Here's how the part is built. I have some questions about the finished solid (model axes, mm). Round coordinates to 2 decimals unless told otherwise and drop trailing zeros. Loops run counter-clockwise (first coordinate to the right, second up) from the corner with the lowest first, then second, coordinate; pieces in that order, holes last. Notation, with made-up numbers: M 86,68 L 99,68 A18 ccw 99,103 Z; hole C -23.75,-33.5 d5. An arc over 180 degrees is marked long. One line per question, with ' | ' between items. Start each with the question number.
```python
from build123d import *

# Parameters (mm, degrees)
SKETCH3_R           = 1.4224
SKETCH3_W           = 6.35
SKETCH3_H           = 6.35
SKETCH3_W_2         = 11.938
SKETCH3_H_2         = 23.114
SKETCH3_W_3         = 101.6
SKETCH3_H_3         = 76.2
BOSS_EXTRUDE1_DEPTH = 6.35
FILLET1_R           = 10.16
FILLET2_R           = 27.94


with BuildPart() as part:
    # Sketch3 → Boss-Extrude1 (new body)
    with BuildSketch(Plane(origin=(0, 0, 0), x_dir=(1, 0, 0), z_dir=(0, 1, 0))):
        with BuildLine():
            Line((182.88, 0), (0, 0))
            Line((0, 0), (0, 262.339276313))
            Line((0, 262.339276313), (182.88, 262.339276313))
            Line((182.88, 262.339276313), (182.88, 169.269638157))
            ThreePointArc((182.88, 169.269638157), (144.78, 131.169638157), (182.88, 93.069638157))
            Line((182.88, 93.069638157), (182.88, 0))
        make_face()
        with Locations(Location((57.15, 38.1, 0), (0, 0, 270))):
            Circle(SKETCH3_R, mode=Mode.SUBTRACT)
        with Locations(Location((57.15, 114.3, 0), (0, 0, 270))):
            Circle(SKETCH3_R, mode=Mode.SUBTRACT)
        with Locations(Location((125.73, 38.1, 0), (0, 0, 90))):
            Circle(SKETCH3_R, mode=Mode.SUBTRACT)
        with Locations(Location((69.85, 151.157668748, 0), (0, 0, 270))):
            Circle(SKETCH3_R, mode=Mode.SUBTRACT)
        with Locations(Location((69.85, 219.737668748, 0), (0, 0, 270))):
            Circle(SKETCH3_R, mode=Mode.SUBTRACT)
        with Locations(Location((113.03, 151.157668748, 0), (0, 0, 90))):
            Circle(SKETCH3_R, mode=Mode.SUBTRACT)
        with Locations(Location((113.03, 219.737668748, 0), (0, 0, 90))):
            Circle(SKETCH3_R, mode=Mode.SUBTRACT)
        with Locations(Location((113.03, 42.601607565, 0), (0, 0, 270))):
            Circle(SKETCH3_R, mode=Mode.SUBTRACT)
        with Locations(Location((113.03, 111.181607565, 0), (0, 0, 270))):
            Circle(SKETCH3_R, mode=Mode.SUBTRACT)
        with Locations(Location((69.85, 111.181607565, 0), (0, 0, 90))):
            Circle(SKETCH3_R, mode=Mode.SUBTRACT)
        with Locations(Location((69.85, 42.601607565, 0), (0, 0, 90))):
            Circle(SKETCH3_R, mode=Mode.SUBTRACT)
        with Locations(Location((125.73, 224.239276313, 0), (0, 0, 270))):
            Circle(SKETCH3_R, mode=Mode.SUBTRACT)
        with Locations(Location((57.15, 224.239276313, 0), (0, 0, 90))):
            Circle(SKETCH3_R, mode=Mode.SUBTRACT)
        with Locations(Location((57.15, 148.039276313, 0), (0, 0, 90))):
            Circle(SKETCH3_R, mode=Mode.SUBTRACT)
        with Locations((22.225, 13.212735966)):
            Rectangle(SKETCH3_W, SKETCH3_H, mode=Mode.SUBTRACT)
        with Locations((160.655, 13.212735966)):
            Rectangle(SKETCH3_W, SKETCH3_H, mode=Mode.SUBTRACT)
        with Locations((160.655, 249.126540348)):
            Rectangle(SKETCH3_W, SKETCH3_H, mode=Mode.SUBTRACT)
        with Locations((22.225, 249.126540348)):
            Rectangle(SKETCH3_W, SKETCH3_H, mode=Mode.SUBTRACT)
        with Locations((166.751, 193.526638157)):
            Rectangle(SKETCH3_W_2, SKETCH3_H_2, mode=Mode.SUBTRACT)
        with Locations((166.751, 68.812638157)):
            Rectangle(SKETCH3_W_2, SKETCH3_H_2, mode=Mode.SUBTRACT)
        with Locations((91.44, 249.126540348)):
            Rectangle(SKETCH3_W_3, SKETCH3_H, mode=Mode.SUBTRACT)
        with Locations((91.44, 13.212735966)):
            Rectangle(SKETCH3_W_3, SKETCH3_H, mode=Mode.SUBTRACT)
        with Locations((123.825, 131.169638157)):
            Rectangle(SKETCH3_W, SKETCH3_H_3, mode=Mode.SUBTRACT)
        with Locations((22.225, 131.169638157)):
            Rectangle(SKETCH3_W, SKETCH3_H_3, mode=Mode.SUBTRACT)
        with Locations((91.44, 42.57414812)):
            Rectangle(SKETCH3_W_2, SKETCH3_H_2, mode=Mode.SUBTRACT)
        with Locations((91.44, 219.765128193)):
            Rectangle(SKETCH3_W_2, SKETCH3_H_2, mode=Mode.SUBTRACT)
    extrude(amount=BOSS_EXTRUDE1_DEPTH)

    # Fillet1
    fillet1_edges = [part.edges().sort_by_distance(p)[0] for p in [
        (0, 3.175, -262.339276313),
        (182.88, 3.175, -262.339276313),
        (182.88, 3.175, 0),
        (0, 3.175, 0),
    ]]
    fillet(fillet1_edges, radius=FILLET1_R)

    # Fillet2
    fillet2_edges = [part.edges().sort_by_distance(p)[0] for p in [
        (182.88, 3.175, -169.269638157),
        (182.88, 3.175, -93.069638157),
    ]]
    fillet(fillet2_edges, radius=FILLET2_R)


solid = part.part
```
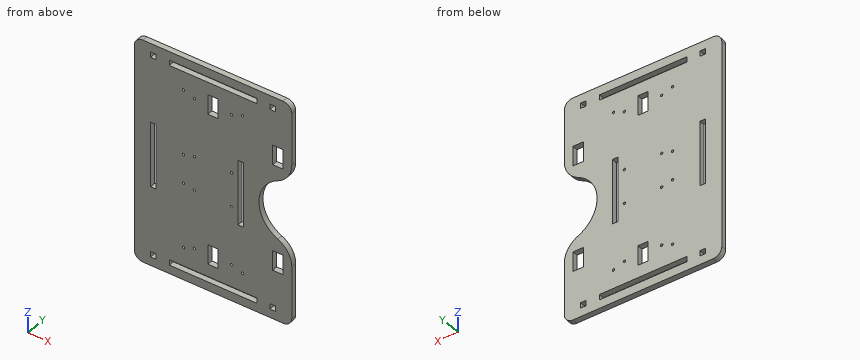
1) Imagine slicing it at D-D (y = 3.75). State how many separate pieces and enclosed holes the cut face has, then the cut area to 3 significant figures.
2) Imagine slicing it at A-A (x = 133). Write out the boundary of the cut face in (y, z).
3) Imagine slicing it at B-B (z = -34). Write out the boundary of the cut face in (x, y).
4) Please list where these lines run through material, in increasing order: L1, parallel to Z at x = 60, y = 2.5; L2, parallel to X at y = 1.5, z = -38.1; L3, parallel to Z at x = 90, y = 2.25. Write a range as from..to.
5) Imagine slicing it at C-C (z = -122). Write out the boundary of the cut face in (x, y), then the cut area to 3 significant figures.
Results are:
1) separate pieces: 1 | enclosed holes: 26 | area: 41,800 mm²
2) outline: M 0,-262.34 L 6.35,-262.34 L 6.35,-252.3 L 0,-252.3 Z; M 0,-245.95 L 6.35,-245.95 L 6.35,-16.39 L 0,-16.39 Z; M 0,-10.04 L 6.35,-10.04 L 6.35,0 L 0,0 Z
3) outline: M 0,0 L 85.47,0 L 85.47,6.35 L 0,6.35 Z; M 97.41,0 L 182.88,0 L 182.88,6.35 L 97.41,6.35 Z
4) L1: -262.34..-252.3, -245.95..-16.39, -10.04..0 | L2: 0..55.73, 58.57..85.47, 97.41..124.31, 127.15..182.88 | L3: -262.34..-252.3, -245.95..-231.32, -208.21..-54.13, -31.02..-16.39, -10.04..0
5) outline: M 0,0 L 19.05,0 L 19.05,6.35 L 0,6.35 Z; M 25.4,0 L 120.65,0 L 120.65,6.35 L 25.4,6.35 Z; M 127,0 L 145.9,0 L 145.9,6.35 L 127,6.35 Z | area: 846 mm²
